Drawing for the job (mm, zero at the part's lowest x, y, z). A direction names the side the tool comes from. Give positions to 0.01 mm unless a question says otherwise; leave off trailing zeros. Write each loop counter-clockwise with the first axis right and the second up, starting at its lowest first coordinate (ties: lowest second). Pieces come first, ordered by that corner, then holes.
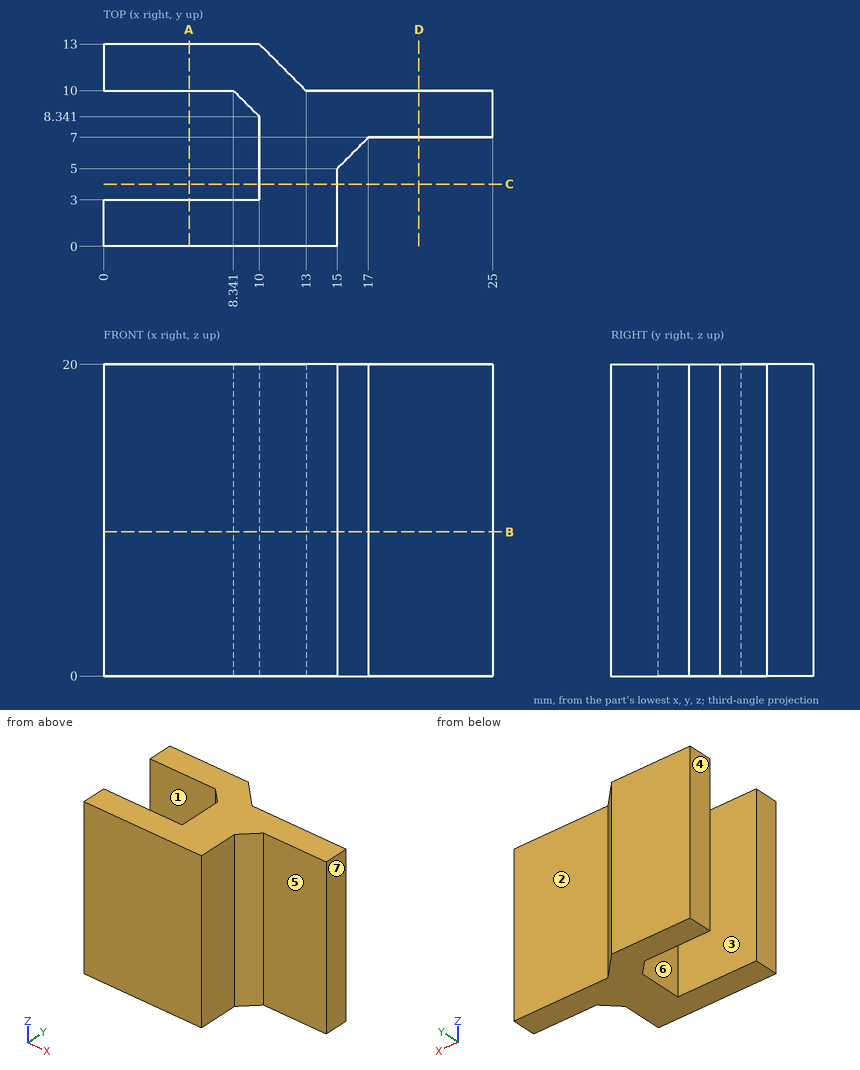
1. Pull direction Y, two halves, no side cores. Call the marked faces 1, 2, 3 and 4: +Y half, -Y half, draft (parallel to the pull), parting line (faces both ways), or undercut.
Calculated:
face 1: undercut
face 2: +Y half
face 3: undercut
face 4: draft
2. Slice it at B-B, the plane z = 9.25. Write the cut outline in (x, y).
Calculated:
outline: (0, 0) - (15, 0) - (15, 5) - (17, 7) - (25, 7) - (25, 10) - (13, 10) - (10, 13) - (0, 13) - (0, 10) - (8.34, 10) - (10, 8.34) - (10, 3) - (0, 3) - close
3. Slice it at D-D, the plane x = 20.25. Write the cut outline in (y, z).
Calculated:
outline: (7, 0) - (10, 0) - (10, 20) - (7, 20) - close
4. Slice it at C-C, the plane y = 4. Write the cut outline in (x, z), and give its area (3 significant figures).
Calculated:
outline: (10, 0) - (15, 0) - (15, 20) - (10, 20) - close
area: 100 mm2
5. Probe probe 1 along Y at (x, z) = (6.5, 6.5); probe 2 along X at (y, z) = (2.25, 8.5); probe 3 along Y at (x, z) = (13.75, 4.5). List the from-to ranges inside material, lowest first.
Calculated:
probe 1: y = 0 to 3, 10 to 13
probe 2: x = 0 to 15
probe 3: y = 0 to 10
6. Slice it at A-A, the plane x = 5.5. Write the cut outline in (y, z), and give its area (3 significant figures).
Calculated:
outline: (0, 0) - (3, 0) - (3, 20) - (0, 20) - close; (10, 0) - (13, 0) - (13, 20) - (10, 20) - close
area: 120 mm2
7. Which spindle directions (+Z, -Z, +X, -X, +Y, -Y) get a long thin tool onto all of the face, cutting with end or side? Do the marked faces 5, 6 and 7. Say none if no direction does.
Calculated:
face 5: +Z, -Z, +X, -Y
face 6: +Z, -Z, -X
face 7: +Z, -Z, +X, +Y, -Y
8. Pin check, flat tips, straight feed: P1, Ø10, axis at x = 17, z = 4.5, coming from the -Y side; P2, Ø1.6, axis at y = 4.5, z = 14, coming from the -X side; P3, Ø5.5, axis at y = 3, z = 12.5, coming from the +X side; P4, Ø6.5, axis at x = 20.5, z = 5, coming from the -Y side. Stop position of each tip, or through.
Calculated:
P1: stops at y = 0
P2: stops at x = 10
P3: stops at x = 15.75
P4: stops at y = 7
